from build123d import *

# Parameters (mm, degrees)
SKETCH1_R           = 6
SKETCH1_R_2         = 20
SKETCH1_R_3         = 9.5
BOSS_EXTRUDE1_DEPTH = 26.5


with BuildPart() as part:
    # Sketch1 → Boss-Extrude1 (new body)
    # profile 1 of 3: a face of its own
    with BuildSketch(Plane.XY):
        with BuildLine():
            ThreePointArc((1.31786679, 47.330365488), (-10.725012101, 33.46783769), (-26.134944205, 43.454558949))
            Line((-26.134944205, 43.454558949), (-20, 0))
            ThreePointArc((-20, 0), (0, 20), (20, 0))
            ThreePointArc((20, 0), (14.142135624, -14.142135624), (0, -20))
            Line((0, -20), (62, -20))
            Line((62, -20), (62, -8.5))
            Line((62, -8.5), (40, -8.5))
            ThreePointArc((40, -8.5), (33.5, -2), (40, 4.5))
            Line((40, 4.5), (62, 4.5))
            Line((62, 4.5), (62, 16))
            ThreePointArc((62, 16), (27.367488456, 23.353309282), (1.31786679, 47.330365488))
        make_face()
    # profile 2 of 3: a face of its own
    with BuildSketch(Plane.XY):
        with BuildLine():
            ThreePointArc((1.31786679, 47.330365488), (-12.68213321, 61.330365488), (-26.68213321, 47.330365488))
            Line((-26.68213321, 47.330365488), (-26.134944205, 43.454558949))
            ThreePointArc((-26.134944205, 43.454558949), (-10.725012101, 33.46783769), (1.31786679, 47.330365488))
        make_face()
        with Locations((-12.68213321, 47.330365488)):
            Circle(SKETCH1_R, mode=Mode.SUBTRACT)
    # profile 3 of 3: a face of its own
    with BuildSketch(Plane.XY):
        Circle(SKETCH1_R_2)
        Circle(SKETCH1_R_3, mode=Mode.SUBTRACT)
    extrude(amount=BOSS_EXTRUDE1_DEPTH)


solid = part.part
Input: part model. Units: mm. Frame: model coordinates. A direction names the side the tool comes from. Coordinates: 2 decimals unless noted, no trailing zeros. Loops run counter-clockwise (first coordinate to the right, second up) from the corner with the lowest first, then second, coordinate; pieces in that order, holes last.
Q1. Draft query along X for faces 3 (the face through (-14.297, -13.986, 13.064)), 4 (the face through (51, -8.5, 13)), 5 (the face through (4.38, -8.43, 13.06)). Return one class per face: +X half, -X half, draft (parallel to the pull), parting line (faces both ways), or undercut.
Q2. Material intervals for line 1 (Y direction, x = 0, z = 12.75); line 2 (X direction, y = -1, z = 3.75); line 3 (Y direction, x = 48.5, z = 25), sorted ascending.
Q3. Contact query for flat-ended pins moving along their axis: pin 1 (9.5 mm diameter, centred on x = -12.68, y = 47.33, fed in from +Z); pin 2 (10 mm diameter, centred on y = 21.5, z = 20, fed in from -X); pin 3 (6 mm diameter, centred on y = 28.5, z = 4, fed in from +X); pin 4 (12 mm diameter, centred on x = -14.5, y = 53, fed in from +Z). Output: stop coordinate, or through.
Q4. Cut plane C-C (x = -1.5). Output: boundary loops of the cut face in (y, z).
Q5. Cut plane D-D (y = 20.5). Output: boundary loops of the cut face in (x, z), then the cut area to 3 significant figures.
Q6. Cut plane A-A (z = 12.5). Output: boundary loops of the cut face in (x, y), then the cut area to 3 significant figures.
Q7. Set-up query: faces 1 (the face through (31, -20, 13)), 2 (the face through (51, 4.5, 13)). Return all of +Z, -Z, +X, -X, +Y, -Y with unobstructed straight access to the full face (end or side cutting, diameter ignored); none if empty.
Q8. Cut plane B-B (x = 45.5). Output: boundary loops of the cut face in (y, z).
Working result:
1. face 3: -X half
1. face 4: draft
1. face 5: undercut
2. line 1: y = -20 to -9.5, 9.5 to 53.26
2. line 2: x = -19.97 to -9.45, 9.45 to 33.58
2. line 3: y = -20 to -8.5, 4.5 to 16.58
3. pin 1: passes through
3. pin 2: stops at x = -23.74
3. pin 3: stops at x = 23.52
3. pin 4: stops at z = 26.5
4. outline: (-19.94, 0) - (-9.38, 0) - (-9.38, 26.5) - (-19.94, 26.5) - close; (9.38, 0) - (55.75, 0) - (55.75, 26.5) - (9.38, 26.5) - close
5. outline: (-22.89, 0) - (33.67, 0) - (33.67, 26.5) - (-22.89, 26.5) - close
5. area: 1,500 mm2
6. outline: (-26.68, 47.33) - (-20, 0) arc R20 ccw to (0, -20) - (62, -20) - (62, -8.5) - (40, -8.5) arc R6.5 cw to (40, 4.5) - (62, 4.5) - (62, 16) arc R67 cw to (1.32, 47.33) arc R14 ccw to start; hole circle Ø12 at (-12.68, 47.33); hole circle Ø19 at (0, 0)
6. area: 3,770 mm2
7. face 1: +Z, -Z, +X, -X, -Y
7. face 2: +Z, -Z, +X
8. outline: (-20, 0) - (-8.5, 0) - (-8.5, 26.5) - (-20, 26.5) - close; (4.5, 0) - (17.08, 0) - (17.08, 26.5) - (4.5, 26.5) - close
